Autodesk Inventor part; units mm, degrees
ref_plane "YZ Plane" through (0, 0, 0) normal (1, 0, 0) x (0, 1, 0)
ref_plane "XZ Plane" through (0, 0, 0) normal (0, 1, 0) x (-1, 0, 0)
ref_plane "XY Plane" through (0, 0, 0) normal (0, 0, 1) x (1, 0, 0)
sketch "Sketch1" plane through (0, 0, 0) normal (0, 0, 1) x (1, 0, 0)
  line L0 (130.175, -104.775) -> (-130.175, -104.775)
  line L1 (-130.175, -104.775) -> (-130.175, 104.775)
  line L2 (-130.175, 104.775) -> (130.175, 104.775)
  line L3 (130.175, 104.775) -> (130.175, -104.775)
  line L4 (130.175, -104.775) -> (-130.175, 104.775) construction
  line L5 (-130.175, -104.775) -> (130.175, 104.775) construction
  point P0 (0, 0)
  dimension "d0" = 260.35
  dimension "d1" = 209.55
extrude "Plate1" add sketch "Sketch1" along normal blind 3.175
sketch "Sketch2" plane through (130.175, -101.6, 0) normal (0, -1, 0) x (1, 0, 0)
  line L0 (-260.35, 0) -> (0, 0)
  line L1 (0, 0) -> (0, 25.4)
  line L2 (0, 25.4) -> (-260.35, 25.4)
  line L3 (-260.35, 25.4) -> (-260.35, 0)
edge flange "Flange1" height 25.4 angle 90 thickness 3.175 bend radius 3.175 thickness toward (0, -1, 0) relief tear relief width 3.175 relief depth 1.5875 corner gap 3.175 corner form 2 edges at (0, -104.775, 3.175) (130.175, 0, 3.175) (0, 104.775, 3.175) (-130.175, 0, 3.175) wall of the first edge with corners at (-130.175, -101.6, 0) (130.175, -101.6, 0) (130.175, -101.6, 25.4) (-130.175, -101.6, 25.4)
bend "Bend1"
corner "Corner1"
equation "\"d0\" = MachineMaxLength - 2 * Thickness"
equation "\"d1\" = MachineMaxWidth - 2 * Thickness"
equation "\"d2\" = Thickness"
equation "\"d3\" = BendReliefWidth"
equation "\"d4\" = BendReliefDepth"
equation "\"d5\" = MinimumRemnant"
equation "\"d6\" = TransitionRadius"
equation "\"d9\" = BendRadius"
equation "\"d10\" = CornerReliefSize"
equation "\"d11\" = GapSize"
equation "\"d12\" = JacobiRadiusSize"
equation "\"BendRadius\" = Thickness"
equation "\"BendReliefWidth\" = Thickness"
equation "\"BendReliefDepth\" = 0.5 * Thickness"
equation "\"CornerReliefSize\" = 4 * Thickness"
equation "\"MinimumRemnant\" = 2 * Thickness"
equation "\"TransitionRadius\" = BendRadius"
equation "\"JacobiRadiusSize\" = BendRadius"
equation "\"GapSize\" = Thickness"
equation "\"MachineMaxHeight\" = 539.75"
equation "\"MachineMaxWidth\" = 215.9"
equation "\"MachineMaxLength\" = 266.7"
equation "\"MachineFluidCapacity\" = 25.4"
equation "\"MaxCompressiveCapacity\" = 20320"
equation "\"WashChamberOD\" = 114.3"
equation "\"WashChamberID\" = 101.6"
equation "\"ConduitThickness\" = 152.4"
equation "\"SealedSurfaceOffset\" = 0.15875"
equation "\"StaticORingThickness\" = 4.7625"
properties part number "FrameBase" material "Stainless Steel"
Geometry check sheet. Reference: the model listing, model coordinates, mm. A direction names the side the tool comes from. Round coordinates to 2 decimals unless told otherwise and drop trailing zeros. Loops run counter-clockwise (first coordinate to the right, second up) from the corner with the lowest first, then second, coordinate; pieces in that order, holes last. Notation, with made-up numbers: (-19.5, 85.25) -> (18.5, 85.25) arc R21 cw to (18.5, 123.25) -> close; hole circle Ø3 at (32, -28). An arc over 180 degrees is marked (long way). Answer as a JSON object with one key per item and string values. Group by question number.
Item 1: Release check for a two-part mould opening along Y. For faces 4 (the face through (2, -101.6, 16)), 5 (the face through (-127, -98.425, 3)), 6 (the face through (-2, 101.6, 16)), 7 (the face through (123.825, -102, 3)) record: pulls with the +Y half, pulls with the -Y half, needs draft (parallel to the pull), parting line crosses it, or undercut.
Item 2: Depth check by flat-ended pin: pin 1 Ø3.5 at (y, z) = (103.5, 12) entering from -X; pin 2 Ø1.5 at (x, y) = (-29.5, 44.5) entering from +Z (3 decimals); pin 3 Ø0.5 at (x, y) = (-129, 98.5) entering from -Z. Enter the tip coordinate at first touch or a pass-through.
Item 3: Set-up check for faces 1 (the face through (-2, 1, 3.175)), 2 (the face through (-123.825, 102, 3)), 3 (the face through (123.825, 102, 3)): record each of +Z, -Z, +X, -X, +Y, -Y from which the full face is reachable in a straight line by a thin tool's end or side.
Item 4: Cross-section at B-B, the plane y = -61.5. Record the cut outline in (x, z) (3 decimals).
Item 5: Thickness scan on line 1 along Y through (x, z) = (23.5, 22.75) (3 decimals); line 2 along X through (y, z) = (-36.5, 18.75) (3 decimals); line 3 along Z through (x, y) = (-22.5, 60) (3 decimals). Record the ranges inside material, lowest first.
Item 6: Cross-section at C-C, the plane x = 53. Record the cut outline in (y, z) (3 decimals).
Item 7: Cross-section at A-A, the plane z = 18. Record the cut outline in (x, y) (3 decimals).
Determined:
{
 "1": {"face 4": "undercut", "face 5": "pulls with the -Y half", "face 6": "undercut", "face 7": "needs draft"},
 "2": {"pin 1": "stops at x = -124.75", "pin 2": "stops at z = 3.175", "pin 3": "stops at z = 2.36"},
 "3": {"face 1": "+Z", "face 2": "-Z, -X, +Y", "face 3": "-Z, +X, +Y"},
 "4": {"outline": "(-130.175, 6.35) arc R6.35 ccw to (-123.825, 0) -> (123.825, 0) arc R6.35 ccw to (130.175, 6.35) -> (130.175, 25.4) -> (127, 25.4) -> (127, 6.35) arc R3.175 cw to (123.825, 3.175) -> (-123.825, 3.175) arc R3.175 cw to (-127, 6.35) -> (-127, 25.4) -> (-130.175, 25.4) -> close"},
 "5": {"line 1": "y = -104.775 to -101.6, 101.6 to 104.775", "line 2": "x = -130.175 to -127, 127 to 130.175", "line 3": "z = 0 to 3.175"},
 "6": {"outline": "(-104.775, 6.35) arc R6.35 ccw to (-98.425, 0) -> (98.425, 0) arc R6.35 ccw to (104.775, 6.35) -> (104.775, 25.4) -> (101.6, 25.4) -> (101.6, 6.35) arc R3.175 cw to (98.425, 3.175) -> (-98.425, 3.175) arc R3.175 cw to (-101.6, 6.35) -> (-101.6, 25.4) -> (-104.775, 25.4) -> close"},
 "7": {"outline": "(-130.175, -99.355) -> (-127, -99.355) -> (-127, 99.355) -> (-130.175, 99.355) -> close; (-124.755, -104.775) -> (124.755, -104.775) -> (124.755, -101.6) -> (-124.755, -101.6) -> close; (-124.755, 101.6) -> (124.755, 101.6) -> (124.755, 104.775) -> (-124.755, 104.775) -> close; (127, -99.355) -> (130.175, -99.355) -> (130.175, 99.355) -> (127, 99.355) -> close"}
}
